Verification items for the finished model (mm, model axes). Give positions to 0.01 mm unless a question says otherwise; leave off trailing zeros. Order: outer loops, then holes, each group sorted by start corner. A loop starts at its lowest first (then second) coordinate and runs counter-clockwise, first axis right, second up. Notation, with made-up numbers: (61, 7.25) - (84, 7.25) arc R16 ccw to (84, 15.25) - close; hole circle Ø7 at (-5.75, 5). An arc over 180 degrees is marked (long way). Answer as a JSON object with one key per item and string values. Group by question number.
(1) Section check B-B (z = 2.1). Count the separate pieces of the cut face and the enclosed holes in it, then the cut area to 3 significant figures.
(2) Depth check by flat-ended pin: pin 1 Ø2 at (x, y) = (20.5, -15.5) entering from -Z; pin 2 Ø1.5 at (x, z) = (-9, 2.5) entering from -Y. Enter the tip coordinate at first touch or a pass-through.
(3) Thickness scan on line 1 (Y direction, x = 11.5, z = 0.75); line 2 (X direction, y = -20.5, z = 2.3); line 3 (Y direction, x = 12.5, z = 2.1). Record the ranges inside material, lowest first.
(4) Section check A-A (y = -17.78). Record the boundary of the cut face in (x, z), then the cut area to 3 significant figures.
```python
from build123d import *

# Parameters (mm, degrees)
F0_R     = 3.175
F0_R_2   = 5
F1_DEPTH = 3


with BuildPart() as f1:
    # F0 (on Top) → F1 (new body)
    with BuildSketch(Plane.XY):
        with BuildLine():
            ThreePointArc((30.955638, -1.657848), (30.988908, -0.829221), (31, 0))
            ThreePointArc((31, 0), (30.988908, 0.829221), (30.955638, 1.657848))
            ThreePointArc((30.955638, 1.657848), (29.251375, 3.074443), (30.623869, 4.814419))
            ThreePointArc((30.623869, 4.814419), (30.322576, 6.445262), (29.934497, 8.057659))
            ThreePointArc((29.934497, 8.057659), (27.97295, 9.088962), (28.95369, 11.076273))
            ThreePointArc((28.95369, 11.076273), (28.319909, 12.608836), (27.605075, 14.105312))
            ThreePointArc((27.605075, 14.105312), (25.471972, 14.70625), (26.018096, 16.854041))
            ThreePointArc((26.018096, 16.854041), (25.079527, 18.221343), (24.069179, 19.536495))
            ThreePointArc((24.069179, 19.536495), (21.857747, 19.680804), (21.945386, 21.895206))
            ThreePointArc((21.945386, 21.895206), (20.743049, 23.03749), (19.481344, 24.113839))
            ThreePointArc((19.481344, 24.113839), (17.288234, 23.795212), (16.913557, 25.979445))
            ThreePointArc((16.913557, 25.979445), (15.5, 26.846788), (14.042081, 27.637293))
            ThreePointArc((14.042081, 27.637293), (11.963142, 26.869656), (11.142525, 28.928258))
            ThreePointArc((11.142525, 28.928258), (9.579527, 29.482752), (7.989112, 29.952865))
            ThreePointArc((7.989112, 29.952865), (6.115203, 28.769766), (4.884511, 30.612768))
            ThreePointArc((4.884511, 30.612768), (3.240382, 30.830179), (1.58698, 30.959352))
            ThreePointArc((1.58698, 30.959352), (0, 29.4125), (-1.58698, 30.959352))
            ThreePointArc((-1.58698, 30.959352), (-3.240382, 30.830179), (-4.884511, 30.612768))
            ThreePointArc((-4.884511, 30.612768), (-4.864464, 30.468287), (-4.857762, 30.322576))
            ThreePointArc((-4.857762, 30.322576), (-6.259123, 28.746026), (-7.989112, 29.952865))
            ThreePointArc((-7.989112, 29.952865), (-9.579527, 29.482752), (-11.142525, 28.928258))
            ThreePointArc((-11.142525, 28.928258), (-11.051928, 28.630061), (-11.021336, 28.319909))
            ThreePointArc((-11.021336, 28.319909), (-12.258922, 26.771453), (-14.042081, 27.637293))
            ThreePointArc((-14.042081, 27.637293), (-15.5, 26.846788), (-16.913557, 25.979445))
            ThreePointArc((-16.913557, 25.979445), (-16.705383, 25.55072), (-16.633843, 25.079527))
            ThreePointArc((-16.633843, 25.079527), (-17.711488, 23.576129), (-19.481344, 24.113839))
            ThreePointArc((-19.481344, 24.113839), (-20.743049, 23.03749), (-21.945386, 21.895206))
            ThreePointArc((-21.945386, 21.895206), (-21.579088, 21.370122), (-21.44999, 20.743049))
            ThreePointArc((-21.44999, 20.743049), (-22.37328, 19.301181), (-24.069179, 19.536495))
            ThreePointArc((-24.069179, 19.536495), (-25.079527, 18.221343), (-26.018096, 16.854041))
            ThreePointArc((-26.018096, 16.854041), (-25.461922, 16.276083), (-25.259288, 15.5))
            ThreePointArc((-25.259288, 15.5), (-26.0355, 14.13546), (-27.605075, 14.105312))
            ThreePointArc((-27.605075, 14.105312), (-28.319909, 12.608836), (-28.95369, 11.076273))
            ThreePointArc((-28.95369, 11.076273), (-28.186596, 10.496116), (-27.895252, 9.579527))
            ThreePointArc((-27.895252, 9.579527), (-28.533276, 8.307265), (-29.934497, 8.057659))
            ThreePointArc((-29.934497, 8.057659), (-30.322576, 6.445262), (-30.623869, 4.814419))
            ThreePointArc((-30.623869, 4.814419), (-29.636933, 4.287435), (-29.242679, 3.240382))
            ThreePointArc((-29.242679, 3.240382), (-29.752916, 2.074337), (-30.955638, 1.657848))
            ThreePointArc((-30.955638, 1.657848), (-30.988908, 0.829221), (-31, 0))
            ThreePointArc((-31, 0), (-30.988908, -0.829221), (-30.955638, -1.657848))
            ThreePointArc((-30.955638, -1.657848), (-29.752916, -2.074337), (-29.242679, -3.240382))
            ThreePointArc((-29.242679, -3.240382), (-29.636933, -4.287435), (-30.623869, -4.814419))
            ThreePointArc((-30.623869, -4.814419), (-30.322576, -6.445262), (-29.934497, -8.057659))
            ThreePointArc((-29.934497, -8.057659), (-28.533276, -8.307265), (-27.895252, -9.579527))
            ThreePointArc((-27.895252, -9.579527), (-28.186596, -10.496116), (-28.95369, -11.076273))
            ThreePointArc((-28.95369, -11.076273), (-28.319909, -12.608836), (-27.605075, -14.105312))
            ThreePointArc((-27.605075, -14.105312), (-26.0355, -14.13546), (-25.259288, -15.5))
            ThreePointArc((-25.259288, -15.5), (-25.461922, -16.276083), (-26.018096, -16.854041))
            ThreePointArc((-26.018096, -16.854041), (-25.079527, -18.221343), (-24.069179, -19.536495))
            ThreePointArc((-24.069179, -19.536495), (-22.37328, -19.301181), (-21.44999, -20.743049))
            ThreePointArc((-21.44999, -20.743049), (-21.579088, -21.370122), (-21.945386, -21.895206))
            ThreePointArc((-21.945386, -21.895206), (-20.743049, -23.03749), (-19.481344, -24.113839))
            ThreePointArc((-19.481344, -24.113839), (-17.711488, -23.576129), (-16.633843, -25.079527))
            ThreePointArc((-16.633843, -25.079527), (-16.705383, -25.55072), (-16.913557, -25.979445))
            ThreePointArc((-16.913557, -25.979445), (-15.5, -26.846788), (-14.042081, -27.637293))
            ThreePointArc((-14.042081, -27.637293), (-12.258922, -26.771453), (-11.021336, -28.319909))
            ThreePointArc((-11.021336, -28.319909), (-11.051928, -28.630061), (-11.142525, -28.928258))
            ThreePointArc((-11.142525, -28.928258), (-9.579527, -29.482752), (-7.989112, -29.952865))
            ThreePointArc((-7.989112, -29.952865), (-6.259123, -28.746026), (-4.857762, -30.322576))
            ThreePointArc((-4.857762, -30.322576), (-4.864464, -30.468287), (-4.884511, -30.612768))
            ThreePointArc((-4.884511, -30.612768), (-3.240382, -30.830179), (-1.58698, -30.959352))
            ThreePointArc((-1.58698, -30.959352), (0, -29.4125), (1.58698, -30.959352))
            ThreePointArc((1.58698, -30.959352), (3.240382, -30.830179), (4.884511, -30.612768))
            ThreePointArc((4.884511, -30.612768), (6.115203, -28.769766), (7.989112, -29.952865))
            ThreePointArc((7.989112, -29.952865), (9.579527, -29.482752), (11.142525, -28.928258))
            ThreePointArc((11.142525, -28.928258), (11.963142, -26.869656), (14.042081, -27.637293))
            ThreePointArc((14.042081, -27.637293), (15.5, -26.846788), (16.913557, -25.979445))
            ThreePointArc((16.913557, -25.979445), (17.288234, -23.795212), (19.481344, -24.113839))
            ThreePointArc((19.481344, -24.113839), (20.743049, -23.03749), (21.945386, -21.895206))
            ThreePointArc((21.945386, -21.895206), (21.857747, -19.680804), (24.069179, -19.536495))
            ThreePointArc((24.069179, -19.536495), (25.079527, -18.221343), (26.018096, -16.854041))
            ThreePointArc((26.018096, -16.854041), (25.471972, -14.70625), (27.605075, -14.105312))
            ThreePointArc((27.605075, -14.105312), (28.319909, -12.608836), (28.95369, -11.076273))
            ThreePointArc((28.95369, -11.076273), (27.97295, -9.088962), (29.934497, -8.057659))
            ThreePointArc((29.934497, -8.057659), (30.322576, -6.445262), (30.623869, -4.814419))
            ThreePointArc((30.623869, -4.814419), (29.251375, -3.074443), (30.955638, -1.657848))
        make_face()
        with Locations((-11.684, -20.237282)):
            Circle(F0_R, mode=Mode.SUBTRACT)
        with Locations((-15.397932, -8.89)):
            Circle(F0_R_2, mode=Mode.SUBTRACT)
        with Locations((0, -17.78)):
            Circle(F0_R_2, mode=Mode.SUBTRACT)
        with Locations((11.684, -20.237282)):
            Circle(F0_R, mode=Mode.SUBTRACT)
        with Locations((15.397932, -8.89)):
            Circle(F0_R_2, mode=Mode.SUBTRACT)
        with BuildLine():
            ThreePointArc((-20.193, 0), (-23.368, -3.175), (-26.543, 0))
            ThreePointArc((-26.543, 0), (-23.368, 3.175), (-20.193, 0))
        make_face(mode=Mode.SUBTRACT)
        with Locations((-15.397932, 8.89)):
            Circle(F0_R_2, mode=Mode.SUBTRACT)
        with BuildLine():
            ThreePointArc((-8.509, 20.237282), (-8.934369, 18.649782), (-10.0965, 17.487651))
            ThreePointArc((-10.0965, 17.487651), (-14.433631, 21.824782), (-8.509, 20.237282))
        make_face(mode=Mode.SUBTRACT)
        with BuildLine():
            ThreePointArc((6.985, 0), (0, -6.985), (-6.985, 0))
            ThreePointArc((-6.985, 0), (-6.049187, 3.4925), (-3.4925, 6.049187))
            ThreePointArc((-3.4925, 6.049187), (-1.807851, 6.746992), (0, 6.985))
            ThreePointArc((0, 6.985), (4.939141, 4.939141), (6.985, 0))
        make_face(mode=Mode.SUBTRACT)
        with Locations((15.397932, 8.89)):
            Circle(F0_R_2, mode=Mode.SUBTRACT)
        with Locations((23.368, 0)):
            Circle(F0_R, mode=Mode.SUBTRACT)
        with BuildLine():
            ThreePointArc((5, 17.78), (3.535534, 14.244466), (0, 12.78))
            ThreePointArc((0, 12.78), (-3.535534, 21.315534), (5, 17.78))
        make_face(mode=Mode.SUBTRACT)
        with Locations((11.684, 20.237282)):
            Circle(F0_R, mode=Mode.SUBTRACT)
    extrude(amount=F1_DEPTH)


solid = f1.part
```
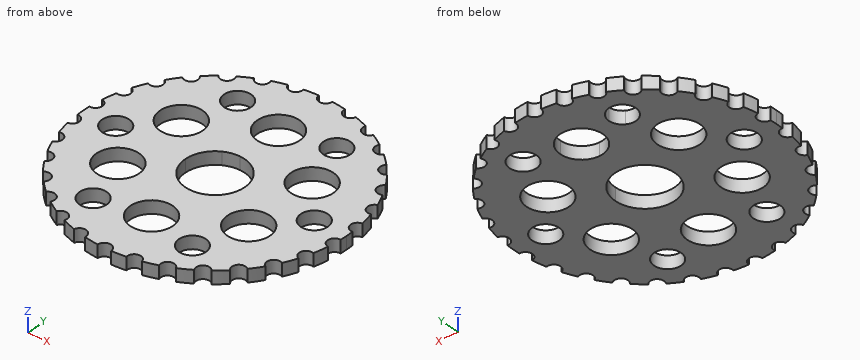
Solutions:
{
 "1": {"separate pieces": "1", "enclosed holes": "13", "area": "2,090 mm2"},
 "2": {"pin 1": "stops at z = 0", "pin 2": "stops at y = -29.88"},
 "3": {"line 1": "y = -27.18 to -23.41, -17.07 to -12.02, -5.76 to 5.76, 12.02 to 17.07, 23.41 to 27.18", "line 2": "x = -21.47 to -14.85, -8.52 to -4.2, 4.2 to 8.52, 14.85 to 21.47", "line 3": "y = -26.74 to -23.31, -17.17 to -12.96, -4.82 to 4.82, 12.96 to 17.17, 23.31 to 26.74"},
 "4": {"outline": "(-25.39, 0) - (-13.69, 0) - (-13.69, 3) - (-25.39, 3) - close; (-9.67, 0) - (-5, 0) - (-5, 3) - (-9.67, 3) - close; (5, 0) - (9.67, 0) - (9.67, 3) - (5, 3) - close; (13.69, 0) - (25.39, 0) - (25.39, 3) - (13.69, 3) - close", "area": "98.2 mm2"}
}
